Part model, mm, in its own coordinate system. Round coordinates to 2 decimals unless told otherwise and drop trailing zeros. Loops run counter-clockwise (first coordinate to the right, second up) from the corner with the lowest first, then second, coordinate; pieces in that order, holes last. Notation, with made-up numbers: M -16.5,71 L -12.5,71 A16 ccw -12.5,80 Z; hole C 87.25,-21.75 d11. An arc over 180 degrees is marked long. Put each result on its own line as item: value. Start each with the question number.
1) Drop a flat-ended pin along its axis: pin 1 Ø12 at (x, z) = (41, 60) entering from +Y. Give the stop position or say it passes through.
2) Slice it at B-B on x = 74. Give the cut face in (y, z).
3) Slice it at C-C on z = 63. Give the cut face in (x, y).
4) Slice it at A-A on y = -0.95. Give the cut face in (x, z), then the cut area to 3 significant figures.
5) Probe line 1 along Z through (x, y) = (66, -0.5); line 2 along X through (y, z) = (-4.1, 49); line 3 along Z through (x, y) = (72, -1.6). List the from-to ranges inside material, lowest first.
```python
from build123d import *

# Parameters (mm, degrees)
F0_W     = 168.040336
F0_H     = 99.579409
F1_DEPTH = 4.572
F2_SIZE2 = 19.064106
F2_SIZE  = 33.02


with BuildPart() as f1:
    # F0 (on Front) → F1 (new body)
    with BuildSketch(Plane.XZ):
        with Locations((0, 23.650117)):
            Rectangle(F0_W, F0_H)
    extrude(amount=F1_DEPTH)

    # F2
    f2_edges = [f1.edges().sort_by_distance(p)[0] for p in [
        (-84.020168, -2.286, 73.439822),
        (84.020168, -2.286, 73.439822),
    ]]
    chamfer(f2_edges, length=F2_SIZE, length2=F2_SIZE2)


solid = f1.part
```
Recorded:
1. pin 1: stops at y = 0
2. outline: M -4.57,-26.14 L 0,-26.14 L 0,57.78 L -4.57,57.78 Z
3. outline: M -70.98,-4.57 L 70.98,-4.57 L 70.98,0 L -70.98,0 Z
4. outline: M -84.02,-26.14 L 84.02,-26.14 L 84.02,40.42 L 64.96,73.44 L -64.96,73.44 L -84.02,40.42 Z
4. area: 16,100 mm2
5. line 1: z = -26.14 to 71.63
5. line 2: x = -79.07 to 79.07
5. line 3: z = -26.14 to 61.24
